The model under review builds one solid part; all positions refer to its coordinate system, in mm. Give positions to 0.01 mm unless a question says otherwise; leave off trailing zeros. Loops run counter-clockwise (first coordinate to the right, second up) from the corner with the lowest first, then second, coordinate; pieces in that order, holes last. Notation, with made-up numbers: (29.25, 51.25) - (73.25, 51.25) arc R14 ccw to (73.25, 62.25) - close; hole circle Ø7 at (24, 51.5). An arc over 180 degrees is marked (long way). Answer as a JSON object with one key per item and string values.
from build123d import *

# Parameters (mm, degrees)
RESSALTO_EXTRUS_O1_DEPTH = 109


with BuildPart() as part:
    # Esboço1 → Ressalto-extrusão1 (new body)
    with BuildSketch(Plane.XY):
        with BuildLine():
            Line((55, -10.355339059), (55, 10.355339059))
            ThreePointArc((55, 10.355339059), (52.716385975, 21.83584203), (46.213203436, 31.568542495))
            Line((46.213203436, 31.568542495), (31.568542495, 46.213203436))
            ThreePointArc((31.568542495, 46.213203436), (21.83584203, 52.716385975), (10.355339059, 55))
            Line((10.355339059, 55), (-10.355339059, 55))
            ThreePointArc((-10.355339059, 55), (-21.83584203, 52.716385975), (-31.568542495, 46.213203436))
            Line((-31.568542495, 46.213203436), (-46.213203436, 31.568542495))
            ThreePointArc((-46.213203436, 31.568542495), (-52.716385975, 21.83584203), (-55, 10.355339059))
            Line((-55, 10.355339059), (-55, -10.355339059))
            ThreePointArc((-55, -10.355339059), (-52.716385975, -21.83584203), (-46.213203436, -31.568542495))
            Line((-46.213203436, -31.568542495), (-31.568542495, -46.213203436))
            ThreePointArc((-31.568542495, -46.213203436), (-21.83584203, -52.716385975), (-10.355339059, -55))
            Line((-10.355339059, -55), (10.355339059, -55))
            ThreePointArc((10.355339059, -55), (21.83584203, -52.716385975), (31.568542495, -46.213203436))
            Line((31.568542495, -46.213203436), (46.213203436, -31.568542495))
            ThreePointArc((46.213203436, -31.568542495), (52.716385975, -21.83584203), (55, -10.355339059))
        make_face()
    extrude(amount=RESSALTO_EXTRUS_O1_DEPTH)


solid = part.part
Q1. Consider section A-A, the plane z = 98. State the section outline as (x, y) points, plus the area to 3 significant figures.
Results:
{"outline": "(-55, -10.36) arc R30 ccw to (-46.21, -31.57) - (-31.57, -46.21) arc R30 ccw to (-10.36, -55) - (10.36, -55) arc R30 ccw to (31.57, -46.21) - (46.21, -31.57) arc R30 ccw to (55, -10.36) - (55, 10.36) arc R30 ccw to (46.21, 31.57) - (31.57, 46.21) arc R30 ccw to (10.36, 55) - (-10.36, 55) arc R30 ccw to (-31.57, 46.21) - (-46.21, 31.57) arc R30 ccw to (-55, 10.36) - close", "area": "9,870 mm^2"}
Q2. To check wall thickness, follow probe 1 along Y at (x, z) = (-10.5, 17); probe 2 along Y at (x, z) = (-42.5, 14.5); probe 3 along X at (y, z) = (-33, 76). State the ranges of each line that lie inside material, in increasing order. Write a range as [from, to].
Results:
{"probe 1": "y = [-55, 55]", "probe 2": "y = [-35.28, 35.28]", "probe 3": "x = [-44.78, 44.78]"}
Q3. Consider section C-C, the plane y = -21. State the section outline as (x, z) points.
Results:
{"outline": "(-53.05, 0) - (53.05, 0) - (53.05, 109) - (-53.05, 109) - close"}
Q4. Clearance check with flat-ended pins moving along their axes: pin 1 Ø1 at (y, z) = (-39, 72) entering from -X; pin 2 Ø1.5 at (x, z) = (-27, 57) entering from +Y; pin 3 Ø5 at (y, z) = (-24, 28.5) entering from +X. State where each tip first meets the part, or that it passes through.
Results:
{"pin 1": "stops at x = -39.28", "pin 2": "stops at y = 50.44", "pin 3": "stops at x = 52.85"}
Q5. The part is to be moulded in two halves that separate along Z. For faces 1 (the face through (-1, 1, 109)), 2 (the face through (52.78, 21.68, 53.74)), 3 (the face through (-1, 1, 0)), say which applies: +Z half, -Z half, draft (parallel to the pull), parting line (faces both ways), or undercut.
Results:
{"face 1": "+Z half", "face 2": "draft", "face 3": "-Z half"}
Q6. Consider section B-B, the plane x = -23.5. State the section outline as (y, z) points, plus the area to 3 significant figures.
Results:
{"outline": "(-51.97, 0) - (51.97, 0) - (51.97, 109) - (-51.97, 109) - close", "area": "11,300 mm^2"}
